```python
from build123d import *

# Parameters (mm, degrees)
SKETCH1_R           = 1.65
SKETCH1_R_2         = 3.75
BOSS_EXTRUDE1_DEPTH = 6.35
FILLET1_R           = 3


with BuildPart() as part:
    # Sketch1 → Boss-Extrude1 (new body)
    with BuildSketch(Plane.XY):
        Polygon((-4, 29.656854249), (29.656854249, -4), (-4, -4), align=None)
        with Locations((0, 20)):
            Circle(SKETCH1_R, mode=Mode.SUBTRACT)
        with Locations((20, 0)):
            Circle(SKETCH1_R, mode=Mode.SUBTRACT)
        Circle(SKETCH1_R, mode=Mode.SUBTRACT)
        with Locations((5.857864376, 5.857864376)):
            Circle(SKETCH1_R_2, mode=Mode.SUBTRACT)
    extrude(amount=BOSS_EXTRUDE1_DEPTH)

    # Fillet1
    fillet1_edges = [part.edges().sort_by_distance(p)[0] for p in [
        (-4, 29.656854249, 3.175),
        (29.656854249, -4, 3.175),
        (-4, -4, 3.175),
    ]]
    fillet(fillet1_edges, radius=FILLET1_R)


solid = part.part
```
Geometry: final body of the model. Coordinates: model frame, mm. Round coordinates to 2 decimals unless told otherwise and drop trailing zeros. Loops run counter-clockwise (first coordinate to the right, second up) from the corner with the lowest first, then second, coordinate; pieces in that order, holes last. Notation, with made-up numbers: (18, 38) -> (37, 38) arc R29 ccw to (37, 71) -> close; hole circle Ø4 at (32.5, -12). An arc over 180 degrees is marked (long way). Write each question's results on one line, items separated by ' | '.
Item 1: Pull-direction query (X, two-part tool) for faces 1 (the face through (11, -4, 3)), 2 (the face through (9.32, 4.42, 3.13)), 3 (the face through (12.665, 12.992, 3.131)); classes: pulls with the +X half, pulls with the -X half, needs draft (parallel to the pull), parting line crosses it, or undercut.
Answers below:
face 1: needs draft | face 2: undercut | face 3: pulls with the +X half
Item 2: Pin query (flat end, axial travel): pin 1 Ø2 at (x, z) = (8.5, 1) entering from +Y; pin 2 Ø4.5 at (x, y) = (5.86, 5.86) entering from -Z; pin 3 Ø3 at (x, z) = (22, 3) entering from +Y. Return the tip coordinate at first contact, or that it passes through.
Answers below:
pin 1: stops at y = 18.16 | pin 2: passes through | pin 3: stops at y = 5.16
Item 3: Cut plane C-C on y = 4. Return the cut outline in (x, z).
Answers below:
outline: (-4, 0) -> (2.6, 0) -> (2.6, 6.35) -> (-4, 6.35) -> close; (9.12, 0) -> (21.66, 0) -> (21.66, 6.35) -> (9.12, 6.35) -> close
Item 4: Cut plane B-B on z = 5. Return the cut outline in (x, y).
Answers below:
outline: (-4, -1) arc R3 ccw to (-1, -4) -> (22.41, -4) arc R3 ccw to (24.54, 1.12) -> (1.12, 24.54) arc R3 ccw to (-4, 22.41) -> close; hole circle Ø3.3 at (0, 0); hole circle Ø3.3 at (0, 20); hole circle Ø7.5 at (5.86, 5.86); hole circle Ø3.3 at (20, 0)
Item 5: Cut plane A-A on x = 7.5. Return the cut outline in (y, z).
Answers below:
outline: (-4, 0) -> (2.49, 0) -> (2.49, 6.35) -> (-4, 6.35) -> close; (9.23, 0) -> (18.16, 0) -> (18.16, 6.35) -> (9.23, 6.35) -> close
Item 6: Line query: probe 1 along Y at (x, z) = (1.5, 6); probe 2 along Y at (x, z) = (0, 3.5); probe 3 along Y at (x, z) = (6.25, 5.25). Output: solid intervals per line, ascending. Write a range as [from, to].
Answers below:
probe 1: y = [-4, -0.69], [0.69, 19.31], [20.69, 24.16] | probe 2: y = [-4, -1.65], [1.65, 18.35], [21.65, 25.24] | probe 3: y = [-4, 2.13], [9.59, 19.41]
Item 7: Cut plane D-D on y = 0. Return the cut outline in (x, z).
Answers below:
outline: (-4, 0) -> (-1.65, 0) -> (-1.65, 6.35) -> (-4, 6.35) -> close; (1.65, 0) -> (18.35, 0) -> (18.35, 6.35) -> (1.65, 6.35) -> close; (21.65, 0) -> (25.24, 0) -> (25.24, 6.35) -> (21.65, 6.35) -> close
